Geometry check sheet. Reference: the model listing, model coordinates, mm. A direction names the side the tool comes from. Round coordinates to 2 decimals unless told otherwise and drop trailing zeros. Write each loop counter-clockwise with the first axis right and the second up, starting at its lowest first coordinate (ties: lowest second). Pieces come first, ordered by that corner, then holes. Notation, with made-up numbers: (12.25, -15.75) - (21.25, -15.75) arc R22 ccw to (21.25, 11.25) - close; hole circle Ø2 at (0, 2). An arc over 180 degrees is marked (long way). Return JSON: item names as keys, results as strings.
```python
from build123d import *

# Parameters (mm, degrees)
SKETCH_1_W          = 32
SKETCH_1_H          = 15
EXTRUDE_1_DEPTH     = 3
SKETCH_2_W          = 32
SKETCH_2_H          = 3
EXTRUDE_2_DEPTH     = 8
SKETCH_3_R          = 1.7
CUT_EXTRUDE_1_DEPTH = 8
CHAMFER_1_SIZE      = 1
FILLET_1_R          = 0.5
FILLET_2_R          = 0.5


with BuildPart() as part:
    # Эскиз1 → Бобышка-Вытянуть1 (new body)
    with BuildSketch(Plane(origin=(0, 0, 0), x_dir=(1, 0, 0), z_dir=(0, 1, 0))):
        Rectangle(SKETCH_1_W, SKETCH_1_H)
    extrude(amount=EXTRUDE_1_DEPTH)

    # Эскиз2 → Бобышка-Вытянуть2 (add)
    with BuildSketch(Plane(origin=(0, 3, 0), x_dir=(1, 0, 0), z_dir=(0, 1, 0))):
        with Locations((0, 6)):
            Rectangle(SKETCH_2_W, SKETCH_2_H)
    extrude(amount=EXTRUDE_2_DEPTH)

    # Эскиз3 → Вырез-Вытянуть1 (cut)
    with BuildSketch(Plane.XZ):
        with Locations(Location((13, 0, 0), (0, 0, 270))):
            Circle(SKETCH_3_R)
        with Locations(Location((-13, 0, 0), (0, 0, 270))):
            Circle(SKETCH_3_R)
    extrude(amount=-CUT_EXTRUDE_1_DEPTH, mode=Mode.SUBTRACT)

    # Фаска1
    # the kernel refuses this chamfer: 1 mm, written as the material it takes off along each edge
    with BuildSketch(Plane(origin=(13, 0, 0), x_dir=(0, 0, -1), z_dir=(-1, 0, 0))) as chamfer_1_piece_1:
        Polygon((1.7 + CHAMFER_1_SIZE, 0), (1.7, -CHAMFER_1_SIZE), (1.7, 0), align=None)
    revolve(axis=Axis((13, 0, 0), (0, -1, 0)), mode=Mode.SUBTRACT)
    with BuildSketch(Plane(origin=(-13, 0, 0), x_dir=(0, 0, -1), z_dir=(-1, 0, 0))) as chamfer_1_piece_2:
        Polygon((1.7 + CHAMFER_1_SIZE, 0), (1.7, -CHAMFER_1_SIZE), (1.7, 0), align=None)
    revolve(axis=Axis((-13, 0, 0), (0, -1, 0)), mode=Mode.SUBTRACT)
    with BuildSketch(Plane(origin=(-18.571682988, 0, 7.5), x_dir=(0, 0.9996219169112968, 0.027495876610586494), z_dir=(1, 0, 0))) as chamfer_1_piece_3:
        Polygon((CHAMFER_1_SIZE * 0.999621916911, -CHAMFER_1_SIZE * 0.0274958766106), (-CHAMFER_1_SIZE * 0.0274958766106, -CHAMFER_1_SIZE * 0.999621916911), (0, 0), align=None)
    extrude(amount=37.143365976, mode=Mode.SUBTRACT)
    with BuildSketch(Plane(origin=(-16, 0, -10.071682988), x_dir=(-0.02749587661058563, 0.9996219169112968, 0), z_dir=(0, 0, 1)), Plane(origin=(16, 0, 10.071682988), x_dir=(0.02749587661058563, 0.9996219169112968, 0), z_dir=(0, 0, -1))) as chamfer_1_piece_4:
        Polygon((CHAMFER_1_SIZE * 0.999621916911, -CHAMFER_1_SIZE * 0.0274958766106), (-CHAMFER_1_SIZE * 0.0274958766106, -CHAMFER_1_SIZE * 0.999621916911), (0, 0), align=None)
    extrude(amount=20.143365976, mode=Mode.SUBTRACT)
    with BuildSketch(Plane(origin=(18.571682988, 0, -7.5), x_dir=(0, -0.027495876610586365, 0.9996219169112968), z_dir=(-1, 0, 0))) as chamfer_1_piece_5:
        Polygon((CHAMFER_1_SIZE * 0.999621916911, CHAMFER_1_SIZE * 0.0274958766106), (-CHAMFER_1_SIZE * 0.0274958766106, CHAMFER_1_SIZE * 0.999621916911), (0, 0), align=None)
    extrude(amount=37.143365976, mode=Mode.SUBTRACT)

    # Скругление1
    # the kernel refuses this fillet: 0.5 mm, written as the material it takes off along each edge
    with BuildSketch(Plane(origin=(-15.5, 10.5, -5), x_dir=(0, 0, 1), z_dir=(0, 1, 0))) as fillet_1_piece_1_section:
        Polygon((0, 0), (FILLET_1_R, 0), (FILLET_1_R, -FILLET_1_R), (0, -FILLET_1_R), align=None)
    fillet_1_piece_1 = extrude(amount=FILLET_1_R, mode=Mode.PRIVATE)
    fillet_1_piece_1 = fillet_1_piece_1 - Plane(origin=(-15.5, 10.5, -5), x_dir=(0.7071067811865475, 0, -0.7071067811865475), z_dir=(0, 1, 0)) * Sphere(FILLET_1_R, mode=Mode.PRIVATE)
    add(fillet_1_piece_1, mode=Mode.SUBTRACT)
    with BuildSketch(Plane(origin=(15.5, 10.5, -5), x_dir=(1, 0, 0), z_dir=(0, 1, 0))) as fillet_1_piece_2_section:
        Polygon((0, 0), (FILLET_1_R, 0), (FILLET_1_R, -FILLET_1_R), (0, -FILLET_1_R), align=None)
    fillet_1_piece_2 = extrude(amount=FILLET_1_R, mode=Mode.PRIVATE)
    fillet_1_piece_2 = fillet_1_piece_2 - Plane(origin=(15.5, 10.5, -5), x_dir=(-0.7071067811865475, 0, -0.7071067811865475), z_dir=(0, 1, 0)) * Sphere(FILLET_1_R, mode=Mode.PRIVATE)
    add(fillet_1_piece_2, mode=Mode.SUBTRACT)
    with BuildSketch(Plane(origin=(-15.5, 10.5, -7), x_dir=(0, 1, 0), z_dir=(0, 0, -1))) as fillet_1_piece_3_section:
        Polygon((0, 0), (FILLET_1_R, 0), (FILLET_1_R, -FILLET_1_R), (0, -FILLET_1_R), align=None)
    fillet_1_piece_3 = extrude(amount=FILLET_1_R, mode=Mode.PRIVATE)
    fillet_1_piece_3 = fillet_1_piece_3 - Plane(origin=(-15.5, 10.5, -7), x_dir=(0.7071067811865475, -0.7071067811865475, 0), z_dir=(0, 0, -1)) * Sphere(FILLET_1_R, mode=Mode.PRIVATE)
    add(fillet_1_piece_3, mode=Mode.SUBTRACT)
    with BuildSketch(Plane(origin=(15.5, 10.5, -7), x_dir=(0, 1, 0), z_dir=(0, 0, -1))) as fillet_1_piece_4_section:
        Polygon((0, 0), (FILLET_1_R, 0), (FILLET_1_R, FILLET_1_R), (0, FILLET_1_R), align=None)
    fillet_1_piece_4 = extrude(amount=FILLET_1_R, mode=Mode.PRIVATE)
    fillet_1_piece_4 = fillet_1_piece_4 - Plane(origin=(15.5, 10.5, -7), x_dir=(-0.7071067811865475, -0.7071067811865475, 0), z_dir=(0, 0, -1)) * Sphere(FILLET_1_R, mode=Mode.PRIVATE)
    add(fillet_1_piece_4, mode=Mode.SUBTRACT)
    with BuildSketch(Plane(origin=(-16, 3, -4.5), x_dir=(1, 0, 0), z_dir=(0, 0, 1))) as fillet_1_piece_5:
        with BuildLine():
            CenterArc((FILLET_1_R, -FILLET_1_R), FILLET_1_R, 90, 90)
            Line((0, -FILLET_1_R), (0, 0))
            Line((0, 0), (FILLET_1_R, 0))
        make_face()
    extrude(amount=13.25, mode=Mode.SUBTRACT)
    with BuildSketch(Plane(origin=(-16, 3, -4.5), x_dir=(0, 0, -1), z_dir=(0, 1, 0))) as fillet_1_piece_6:
        with BuildLine():
            CenterArc((FILLET_1_R, -FILLET_1_R), FILLET_1_R, 90, 90)
            Line((0, -FILLET_1_R), (0, 0))
            Line((0, 0), (FILLET_1_R, 0))
        make_face()
    extrude(amount=7.5, mode=Mode.SUBTRACT)
    with BuildSketch(Plane(origin=(16, 3, -4.5), x_dir=(0, 0, -1), z_dir=(0, 1, 0))) as fillet_1_piece_7:
        with BuildLine():
            CenterArc((FILLET_1_R, FILLET_1_R), FILLET_1_R, 180, 90)
            Line((0, FILLET_1_R), (0, 0))
            Line((0, 0), (FILLET_1_R, 0))
        make_face()
    extrude(amount=7.5, mode=Mode.SUBTRACT)
    with BuildSketch(Plane(origin=(-16, 11, -5), x_dir=(0, -1, 0), z_dir=(0, 0, -1)), Plane(origin=(16, 11, -7), x_dir=(0, -1, 0), z_dir=(0, 0, 1))) as fillet_1_piece_8:
        with BuildLine():
            CenterArc((FILLET_1_R, -FILLET_1_R), FILLET_1_R, 90, 90)
            Line((0, -FILLET_1_R), (0, 0))
            Line((0, 0), (FILLET_1_R, 0))
        make_face()
    extrude(amount=2, mode=Mode.SUBTRACT)
    with BuildSketch(Plane(origin=(15.5, 11, -4.5), x_dir=(0, 0, -1), z_dir=(-1, 0, 0))) as fillet_1_piece_9:
        with BuildLine():
            CenterArc((FILLET_1_R, FILLET_1_R), FILLET_1_R, 180, 90)
            Line((0, FILLET_1_R), (0, 0))
            Line((0, 0), (FILLET_1_R, 0))
        make_face()
    extrude(amount=31, mode=Mode.SUBTRACT)
    with BuildSketch(Plane(origin=(-15.5, 11, -7.5), x_dir=(0, -1, 0), z_dir=(1, 0, 0))) as fillet_1_piece_10:
        with BuildLine():
            CenterArc((FILLET_1_R, -FILLET_1_R), FILLET_1_R, 90, 90)
            Line((0, -FILLET_1_R), (0, 0))
            Line((0, 0), (FILLET_1_R, 0))
        make_face()
    extrude(amount=31, mode=Mode.SUBTRACT)
    with BuildSketch(Plane(origin=(-16, 1, -8.017766953), x_dir=(0, 1, 0), z_dir=(0, 0, 1)), Plane(origin=(16, 1, 8.017766953), x_dir=(0, 1, 0), z_dir=(0, 0, -1))) as fillet_1_piece_11:
        with BuildLine():
            CenterArc((FILLET_1_R * 0.414213562373, -FILLET_1_R), FILLET_1_R, 90, 45)
            Line((-FILLET_1_R * 0.292893218814, -FILLET_1_R * 0.292893218814), (0, 0))
            Line((0, 0), (FILLET_1_R * 0.414213562373, 0))
        make_face()
    extrude(amount=16.035533906, mode=Mode.SUBTRACT)
    with BuildSketch(Plane(origin=(16, 3, 8.75), x_dir=(0, -1, 0), z_dir=(0, 0, -1))) as fillet_1_piece_12:
        with BuildLine():
            CenterArc((FILLET_1_R, FILLET_1_R), FILLET_1_R, 180, 90)
            Line((0, FILLET_1_R), (0, 0))
            Line((0, 0), (FILLET_1_R, 0))
        make_face()
    extrude(amount=13.25, mode=Mode.SUBTRACT)
    with BuildSketch(Plane(origin=(16, -0.25, 7.5), x_dir=(-1, 0, 0), z_dir=(0, 1, 0))) as fillet_1_piece_13:
        with BuildLine():
            CenterArc((FILLET_1_R, -FILLET_1_R), FILLET_1_R, 90, 90)
            Line((0, -FILLET_1_R), (0, 0))
            Line((0, 0), (FILLET_1_R, 0))
        make_face()
    extrude(amount=4.5, mode=Mode.SUBTRACT)
    with BuildSketch(Plane(origin=(-16, -0.25, 7.5), x_dir=(1, 0, 0), z_dir=(0, 1, 0))) as fillet_1_piece_14:
        with BuildLine():
            CenterArc((FILLET_1_R, FILLET_1_R), FILLET_1_R, 180, 90)
            Line((0, FILLET_1_R), (0, 0))
            Line((0, 0), (FILLET_1_R, 0))
        make_face()
    extrude(amount=4.5, mode=Mode.SUBTRACT)
    with BuildSketch(Plane(origin=(-16, 10.5, -7.5), x_dir=(0, 0, 1), z_dir=(0, -1, 0)), Plane(origin=(16, -0.25, -7.5), x_dir=(0, 0, 1), z_dir=(0, 1, 0))) as fillet_1_piece_15:
        with BuildLine():
            CenterArc((FILLET_1_R, -FILLET_1_R), FILLET_1_R, 90, 90)
            Line((0, -FILLET_1_R), (0, 0))
            Line((0, 0), (FILLET_1_R, 0))
        make_face()
    extrude(amount=10.75, mode=Mode.SUBTRACT)
    with BuildSketch(Plane(origin=(-16, 3, -5.75), x_dir=(1, 0, 0), z_dir=(0, 0, 1))) as fillet_1_piece_16a_section:
        with BuildLine():
            CenterArc((FILLET_1_R, -FILLET_1_R), FILLET_1_R, 90, 90)
            Line((0, -FILLET_1_R), (0, 0))
            Line((0, 0), (FILLET_1_R, 0))
        make_face()
    fillet_1_piece_16a = extrude(amount=14.5, mode=Mode.PRIVATE)
    fillet_1_piece_16a = split(fillet_1_piece_16a, bisect_by=Plane(origin=(-15.886802443, 2.886802443, -4.5), z_dir=(0, 0, -1)), keep=Keep.TOP, mode=Mode.PRIVATE)
    with BuildSketch(Plane(origin=(-16, 1.75, -4.5), x_dir=(0, 0, -1), z_dir=(0, 1, 0))) as fillet_1_piece_16b_section:
        with BuildLine():
            CenterArc((FILLET_1_R, -FILLET_1_R), FILLET_1_R, 90, 90)
            Line((0, -FILLET_1_R), (0, 0))
            Line((0, 0), (FILLET_1_R, 0))
        make_face()
    fillet_1_piece_16b = extrude(amount=8.75, mode=Mode.PRIVATE)
    fillet_1_piece_16b = split(fillet_1_piece_16b, bisect_by=Plane(origin=(-15.886802443, 3, -4.613197557), z_dir=(0, -1, 0)), keep=Keep.TOP, mode=Mode.PRIVATE)
    fillet_1_piece_16 = fillet_1_piece_16a & fillet_1_piece_16b
    add(fillet_1_piece_16, mode=Mode.SUBTRACT)
    with BuildSketch(Plane(origin=(16, 1.75, -4.5), x_dir=(0, 0, -1), z_dir=(0, 1, 0))) as fillet_1_piece_17a_section:
        with BuildLine():
            CenterArc((FILLET_1_R, FILLET_1_R), FILLET_1_R, 180, 90)
            Line((0, FILLET_1_R), (0, 0))
            Line((0, 0), (FILLET_1_R, 0))
        make_face()
    fillet_1_piece_17a = extrude(amount=8.75, mode=Mode.PRIVATE)
    fillet_1_piece_17a = split(fillet_1_piece_17a, bisect_by=Plane(origin=(15.886802443, 3, -4.613197557), z_dir=(0, -1, 0)), keep=Keep.TOP, mode=Mode.PRIVATE)
    with BuildSketch(Plane(origin=(16, 3, 8.75), x_dir=(0, -1, 0), z_dir=(0, 0, -1))) as fillet_1_piece_17b_section:
        with BuildLine():
            CenterArc((FILLET_1_R, FILLET_1_R), FILLET_1_R, 180, 90)
            Line((0, FILLET_1_R), (0, 0))
            Line((0, 0), (FILLET_1_R, 0))
        make_face()
    fillet_1_piece_17b = extrude(amount=14.5, mode=Mode.PRIVATE)
    fillet_1_piece_17b = split(fillet_1_piece_17b, bisect_by=Plane(origin=(15.886802443, 2.886802443, -4.5), z_dir=(0, 0, -1)), keep=Keep.TOP, mode=Mode.PRIVATE)
    fillet_1_piece_17 = fillet_1_piece_17a & fillet_1_piece_17b
    add(fillet_1_piece_17, mode=Mode.SUBTRACT)

    # Скругление2
    # the kernel refuses this fillet: 0.5 mm, written as the material it takes off along each edge
    with BuildSketch(Plane(origin=(-15.5, 2.5, 7), x_dir=(0, 1, 0), z_dir=(0, 0, 1))) as fillet_2_piece_1_section:
        Polygon((0, 0), (FILLET_2_R, 0), (FILLET_2_R, FILLET_2_R), (0, FILLET_2_R), align=None)
    fillet_2_piece_1 = extrude(amount=FILLET_2_R, mode=Mode.PRIVATE)
    fillet_2_piece_1 = fillet_2_piece_1 - Plane(origin=(-15.5, 2.5, 7), x_dir=(0.7071067811865475, -0.7071067811865475, 0), z_dir=(0, 0, 1)) * Sphere(FILLET_2_R, mode=Mode.PRIVATE)
    add(fillet_2_piece_1, mode=Mode.SUBTRACT)
    with BuildSketch(Plane(origin=(15.5, 2.5, 7), x_dir=(0, 1, 0), z_dir=(0, 0, 1))) as fillet_2_piece_2_section:
        Polygon((0, 0), (FILLET_2_R, 0), (FILLET_2_R, -FILLET_2_R), (0, -FILLET_2_R), align=None)
    fillet_2_piece_2 = extrude(amount=FILLET_2_R, mode=Mode.PRIVATE)
    fillet_2_piece_2 = fillet_2_piece_2 - Plane(origin=(15.5, 2.5, 7), x_dir=(-0.7071067811865475, -0.7071067811865475, 0), z_dir=(0, 0, 1)) * Sphere(FILLET_2_R, mode=Mode.PRIVATE)
    add(fillet_2_piece_2, mode=Mode.SUBTRACT)
    with BuildSketch(Plane(origin=(-15.5, 3, 7.5), x_dir=(0, -1, 0), z_dir=(1, 0, 0))) as fillet_2_piece_3:
        with BuildLine():
            CenterArc((FILLET_2_R, FILLET_2_R), FILLET_2_R, 180, 90)
            Line((0, FILLET_2_R), (0, 0))
            Line((0, 0), (FILLET_2_R, 0))
        make_face()
    extrude(amount=31, mode=Mode.SUBTRACT)


solid = part.part
```
(1) Section check D-D, the plane y = 7. Enter the section's corners in (x, z).
Response values:
{"outline": "(-16, -7) arc R0.5 ccw to (-15.5, -7.5) - (15.5, -7.5) arc R0.5 ccw to (16, -7) - (16, -5) arc R0.5 ccw to (15.5, -4.5) - (-15.5, -4.5) arc R0.5 ccw to (-16, -5) - close"}
(2) Material ranges on line 1 along X through (y, z) = (1.45, 0); line 2 along Y through (x, z) = (-9.5, 3); line 3 along Z through (x, y) = (-3, 7.75), recorded low to high. Write a range as [from, to].
Response values:
{"line 1": "x = [-16, -14.7], [-11.3, 11.3], [14.7, 16]", "line 2": "y = [0, 3]", "line 3": "z = [-7.5, -4.5]"}
(3) Release check for a two-part mould opening along X. For faces 1 (the face through (0.2, 0.5, -7)), 2 (the face through (15.5, 0.5, 0.1)), 3 (the face through (-11.156, 0.84, 0.242)) record: pulls with the +X half, pulls with the -X half, needs draft (parallel to the pull), parting line crosses it, or undercut.
Response values:
{"face 1": "needs draft", "face 2": "pulls with the +X half", "face 3": "undercut"}
(4) Section check B-B, the plane x = 13. Enter the section's corners in (y, z).
Response values:
{"outline": "(0, -6.5) - (1, -7.5) - (10.5, -7.5) arc R0.5 ccw to (11, -7) - (11, -5) arc R0.5 ccw to (10.5, -4.5) - (3, -4.5) - (3, -1.7) - (1, -1.7) - (0, -2.7) - close; (0, 2.7) - (1, 1.7) - (3, 1.7) - (3, 7) arc R0.5 ccw to (2.5, 7.5) - (1, 7.5) - (0, 6.5) - close"}
(5) Section check C-C, the plane x = -1. Enter the section's corners in (y, z).
Response values:
{"outline": "(0, -6.5) - (1, -7.5) - (10.5, -7.5) arc R0.5 ccw to (11, -7) - (11, -5) arc R0.5 ccw to (10.5, -4.5) - (3, -4.5) - (3, 7) arc R0.5 ccw to (2.5, 7.5) - (1, 7.5) - (0, 6.5) - close"}
(6) Gauge pin test, flat ends, axial feed: pin 1 (6 mm diameter, centred on x = -5, z = -0.5, fed in from +Y); pin 2 (2.5 mm diameter, centred on x = -13, z = 0, fed in from -Y). Record the tip position at first contact, or that the pin passes through.
Response values:
{"pin 1": "stops at y = 3", "pin 2": "passes through"}
(7) Access from +Z, -Z, +X, -X, +Y, -Y to the whole of each face (thin tool, end or side, straight path). Record for faces 4 (the face through (0, 11, -6)), 5 (the face through (0, 3, 1)).
Response values:
{"face 4": "+Z, -Z, +X, -X, +Y", "face 5": "+Z, +X, -X, +Y"}
(8) Section check A-A, the plane z = 0. Enter the section's corners in (x, y), plus the area to 3 significant figures.
Response values:
{"outline": "(-16, 1.21) arc R0.5 ccw to (-15.85, 0.85) - (-15.35, 0.35) - (-14.7, 1) - (-14.7, 3) - (-15.5, 3) arc R0.5 ccw to (-16, 2.5) - close; (-11.3, 1) - (-10.3, 0) - (10.3, 0) - (11.3, 1) - (11.3, 3) - (-11.3, 3) - close; (14.7, 1) - (15.35, 0.35) - (15.85, 0.85) arc R0.5 ccw to (16, 1.21) - (16, 2.5) arc R0.5 ccw to (15.5, 3) - (14.7, 3) - close", "area": "72.7 mm^2"}
